from build123d import *

# Parameters (mm, degrees)
F1_DEPTH = 22.606
F2_R     = 1.8288
F3_DEPTH = 25.4
F4_R     = 0.79375
F5_DEPTH = 9.0530042065


with BuildPart() as f1:
    # F0 (on Top) → F1 (new body)
    with BuildSketch(Plane.XY):
        with BuildLine():
            ThreePointArc((0, 25.4), (5.2044977798, 12.7), (0, 0))
            Line((0, 0), (13.2400867088, 0))
            Line((13.2400867088, 0), (13.2400867088, 25.4))
            Line((13.2400867088, 25.4), (0, 25.4))
        make_face()
    extrude(amount=F1_DEPTH)

    # F2 (on face) → F3 (cut, through all)
    with BuildSketch(Plane(origin=(0, 25.4, 0), x_dir=(-1, 0, 0), z_dir=(0, 1, 0))):
        with Locations((-9.2713367088, 3.96875)):
            Circle(F2_R)
        with Locations((-9.2713367088, 18.63725)):
            Circle(F2_R)
    extrude(amount=-F3_DEPTH, mode=Mode.SUBTRACT)

    # F4 (on face) → F5 (cut, up to face)
    with BuildSketch(Plane.YZ.offset(13.2400867088)):
        with Locations((12.7, 11.303)):
            Circle(F4_R)
    extrude(amount=-F5_DEPTH, mode=Mode.SUBTRACT)


solid = f1.part
Design review of the part built by this model. Coordinates are the model's own, in mm. Give positions to 0.01 mm unless a question says otherwise; leave off trailing zeros. Loops run counter-clockwise (first coordinate to the right, second up) from the corner with the lowest first, then second, coordinate; pieces in that order, holes last. Notation, with made-up numbers: (40.25, 46) -> (85.25, 46) arc R6 ccw to (85.25, 52) -> close; hole circle Ø9 at (77.5, 71). An arc over 180 degrees is marked (long way). One line per question, with ' | ' between items. Start each with the question number.
(1) Insertion check: P1, Ø12, axis at y = 8, z = 19, coming from the -X side; P2, Ø10, axis at y = 11.5, z = 12, coming from the -X side; P3, Ø4, axis at y = 16.5, z = 16.5, coming from the -X side. Each pin has a flat end and moves straight along its axis. Give the tip position at first contact, or say it passes through.
(2) We need section C-C (x = 3.25). State the section outline as (y, z) points.
(3) We need section A-A (x = 8). State the section outline as (y, z) points, and give its area (3 significant figures).
(4) Draft analysis for pull direction Z (two halves, no side actions). For faces 1 (the face through (9.27, 13.07, 10.6)), 2 (the face through (8, 13, 22.606)), 3 (the face through (7, 25.4, 11)), 4 (the face through (10.619, 12.878, 5.205)), state which applies: +Z half, -Z half, draft (parallel to the pull), parting line (faces both ways), or undercut.
(5) We need section B-B (y = 12.7). State the section outline as (x, z) points.
(6) We need section D-D (z = 4.5). State the section outline as (x, y) points (1 decimal), and give its area (3 significant figures).
(7) For line 1 (Z direction, x = 9.25, y = 11.75); line 2 (Z direction, x = 10.5, y = 3.25); line 3 (X direction, y = 23.25, z = 2.5), list the stretches that pass through material, from the lowest coordinate up.
The answers:
1) P1: stops at x = 1.7 | P2: stops at x = 4.11 | P3: stops at x = 4.25
2) outline: (0, 0) -> (4.52, 0) -> (4.52, 22.61) -> (0, 22.61) -> close; (20.88, 0) -> (25.4, 0) -> (25.4, 22.61) -> (20.88, 22.61) -> close
3) outline: (0, 0) -> (25.4, 0) -> (25.4, 2.65) -> (0, 2.65) -> close; (0, 5.28) -> (25.4, 5.28) -> (25.4, 17.32) -> (0, 17.32) -> close; (0, 19.95) -> (25.4, 19.95) -> (25.4, 22.61) -> (0, 22.61) -> close; hole circle Ø1.59 at (12.7, 11.3) | area: 439 mm^2
4) face 1: undercut | face 2: +Z half | face 3: draft | face 4: undercut
5) outline: (5.2, 0) -> (13.24, 0) -> (13.24, 10.51) -> (5.2, 10.51) -> close; (5.2, 12.1) -> (13.24, 12.1) -> (13.24, 22.61) -> (5.2, 22.61) -> close; hole circle Ø3.66 at (9.27, 3.97); hole circle Ø3.66 at (9.27, 18.64)
6) outline: (0, 0) -> (7.5, 0) -> (7.5, 25.4) -> (0, 25.4) arc R18.1 cw to start; (11, 0) -> (13.2, 0) -> (13.2, 25.4) -> (11, 25.4) -> close | area: 156 mm^2
7) line 1: z = 0 to 2.14, 5.8 to 16.81, 20.47 to 22.61 | line 2: z = 0 to 2.61, 5.32 to 17.28, 19.99 to 22.61 | line 3: x = 1.81 to 8.18, 10.36 to 13.24
